The model under review builds one solid part; all positions refer to its coordinate system, in mm. Coordinates: 2 decimals unless noted, no trailing zeros. Write each loop counter-clockwise with the first axis right and the second up, starting at its lowest first coordinate (ties: lowest second). Pieces come first, ordered by that corner, then holes.
```python
from build123d import *

# Parameters (mm, degrees)
ESBO_O1_R                = 10
ESBO_O1_R_2              = 5.05
RESSALTO_EXTRUS_O1_DEPTH = 5.175
CHANFRO1_SIZE            = 0.5


with BuildPart() as part:
    # Esboço1 → Ressalto-extrusão1 (new, symmetric)
    with BuildSketch(Plane.XY):
        Circle(ESBO_O1_R)
        Circle(ESBO_O1_R_2, mode=Mode.SUBTRACT)
    extrude(amount=RESSALTO_EXTRUS_O1_DEPTH, both=True)

    # Chanfro1
    chanfro1_edges = [part.edges().sort_by_distance(p)[0] for p in [
        (-10, 0, -5.175),
        (-10, 0, 5.175),
        (-5.05, 0, -5.175),
        (-5.05, 0, 5.175),
    ]]
    chamfer(chanfro1_edges, length=CHANFRO1_SIZE)


solid = part.part
```
Item 1: For pin 1 (5 mm diameter, centred on x = -6, z = 1, fed in from -Y); pin 2 (1.5 mm diameter, centred on y = 5, z = 1, fed in from +X), all flat-tipped, find the tip position at first contact; note any pin that passes through.
Solved:
pin 1: stops at y = -9.37
pin 2: stops at x = 9.05
Item 2: Mouldability with a two-part tool opening along X and no side actions: class faces 1 (the face through (-2.17, -9.76, 0.07)), 2 (the face through (4.1, -4.1, -5.175)), 3 (the face through (4.817, 1.517, -0.065)) as pulls with the +X half, pulls with the -X half, needs draft (parallel to the pull), parting line crosses it, or undercut.
Solved:
face 1: parting line crosses it
face 2: needs draft
face 3: undercut
Item 3: Take a section at A-A, the plane x = 0. Write out the cut boundary in (y, z) (3 decimals).
Solved:
outline: (-10, -4.675) - (-9.5, -5.175) - (-5.55, -5.175) - (-5.05, -4.675) - (-5.05, 4.675) - (-5.55, 5.175) - (-9.5, 5.175) - (-10, 4.675) - close; (5.05, -4.675) - (5.55, -5.175) - (9.5, -5.175) - (10, -4.675) - (10, 4.675) - (9.5, 5.175) - (5.55, 5.175) - (5.05, 4.675) - close
Item 4: To check wall thickness, follow line 1 along Y through (x, z) = (0, -2.25); line 2 along X through (y, z) = (-3.75, 3.75); line 3 along Y through (x, z) = (3, -2.75). State the ranges of each line that lie inside material, in increasing order.
Solved:
line 1: y = -10 to -5.05, 5.05 to 10
line 2: x = -9.27 to -3.38, 3.38 to 9.27
line 3: y = -9.54 to -4.06, 4.06 to 9.54
Item 5: Take a section at C-C, the plane z = -1.5. Write out the cut boundary in (x, y).
Solved:
outline: circle Ø20 at (0, 0); hole circle Ø10.1 at (0, 0)
